Geometry check sheet. Reference: the model listing, model coordinates, mm. Face numbers are marked on the shaded views. A direction names the side the tool comes from. Coordinates: 2 decimals unless noted, no trailing zeros. Loops run counter-clockwise (first coordinate to the right, second up) from the corner with the lowest first, then second, coordinate; pieces in that order, holes last.
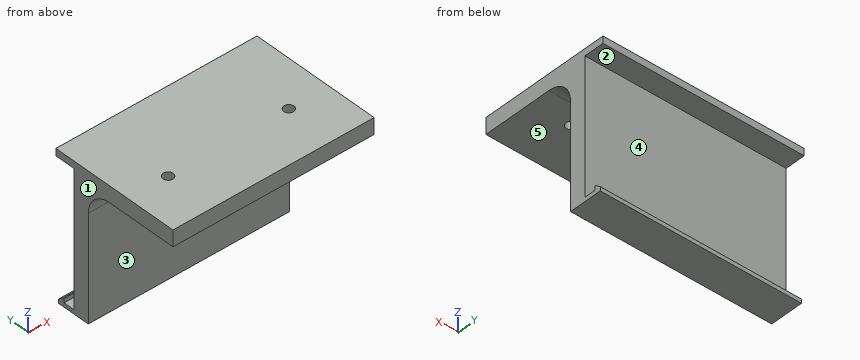
from build123d import *

# Parameters (mm, degrees)
F1_DEPTH = 50
F3_DEPTH = 100
F4_R     = 2.5
F5_DEPTH = 8
F6_R     = 12


with BuildPart() as f1:
    # F0 (on Right) → F1 (new body, symmetric)
    with BuildSketch(Plane.YZ):
        Polygon((0, -3.5), (0, 0), (-65, 0), (-65, -8), (-18, -8), (-18, -72.5), (-1.5, -72.5), (-1.5, -68.5), (-4.5, -68.5), (-4.5, -70.5), (-10, -70.5), (-10, -3.5), align=None)
    extrude(amount=F1_DEPTH, both=True)

    # F2 (on face) → F3 (cut, through all)
    with BuildSketch(Plane.YZ.offset(50)):
        Polygon((-1.5, -68.5), (-4, -68.5), (-1.5, -70.5), align=None)
    extrude(amount=-F3_DEPTH, mode=Mode.SUBTRACT)

    # F4 (on face) → F5 (cut, through all)
    with BuildSketch(Plane.XY):
        with Locations((-30, -40)):
            Circle(F4_R)
        with Locations((30, -40)):
            Circle(F4_R)
    extrude(amount=-F5_DEPTH, mode=Mode.SUBTRACT)

    # F6
    f6_edges = [f1.edges().sort_by_distance(p)[0] for p in [
        (0, -18, -8),
    ]]
    fillet(f6_edges, radius=F6_R)


solid = f1.part
1) Depth check by flat-ended pin: pin 1 (8 mm diameter, centred on x = -30, y = -40, fed in from -Z); pin 2 (3 mm diameter, centred on x = -28.5, z = -45, fed in from -Y); pin 3 (1.6 mm diameter, centred on x = 12, z = -71.5, fed in from +Y). Enter the tip coordinate at first touch or a pass-through.
Data:
pin 1: stops at z = -8
pin 2: stops at y = -18
pin 3: stops at y = -1.5
2) Mould release check, pull along Z, two halves, no side actions. Record for the marked faces 3, 4 and 5: +Z half, -Z half, draft (parallel to the pull), parting line (faces both ways), or undercut.
Data:
face 3: draft
face 4: undercut
face 5: -Z half
3) Section check A-A on x = 30. Record the cut outline in (y, z), and give its area (3 significant figures).
Data:
outline: (-65, -8) - (-42.5, -8) - (-42.5, 0) - (-65, 0) - close; (-37.5, -8) - (-30, -8) arc R12 cw to (-18, -20) - (-18, -72.5) - (-1.5, -72.5) - (-1.5, -70.5) - (-4, -68.5) - (-4.5, -68.5) - (-4.5, -70.5) - (-10, -70.5) - (-10, -3.5) - (0, -3.5) - (0, 0) - (-37.5, 0) - close
area: 1,000 mm2
4) Section check B-B on y = -40. Record the cut outline in (x, z), and give its area (3 significant figures).
Data:
outline: (-50, -8) - (-32.5, -8) - (-32.5, 0) - (-50, 0) - close; (-27.5, -8) - (27.5, -8) - (27.5, 0) - (-27.5, 0) - close; (32.5, -8) - (50, -8) - (50, 0) - (32.5, 0) - close
area: 720 mm2
5) Access from +Z, -Z, +X, -X, +Y, -Y to the whole of each face (thin tool, end or side, straight path). Record for the marked faces 1 and 2.
Data:
face 1: +Z, -Z, -X, +Y, -Y
face 2: +X, -X, +Y
6) Material ranges on probe 1 along Y at (x, z) = (-30, -6); probe 2 along Y at (x, z) = (-30, -3); probe 3 along Z at (x, y) = (-44.5, -8), recorded low to high.
Data:
probe 1: y = -65 to -42.5, -37.5 to -10
probe 2: y = -65 to -42.5, -37.5 to 0
probe 3: z = -72.5 to -70.5, -3.5 to 0
7) Section check D-D on y = -60. Record the cut outline in (x, z), and give its area (3 significant figures).
Data:
outline: (-50, -8) - (50, -8) - (50, 0) - (-50, 0) - close
area: 800 mm2
8) Section check C-C on x = -20.5. Record the cut outline in (y, z).
Data:
outline: (-65, -8) - (-30, -8) arc R12 cw to (-18, -20) - (-18, -72.5) - (-1.5, -72.5) - (-1.5, -70.5) - (-4, -68.5) - (-4.5, -68.5) - (-4.5, -70.5) - (-10, -70.5) - (-10, -3.5) - (0, -3.5) - (0, 0) - (-65, 0) - close
